Input: part model. Units: mm. Frame: model coordinates. Face numbers are marked on the shaded views. A direction names the side the tool comes from. Round coordinates to 2 decimals unless told otherwise and drop trailing zeros. Write each loop counter-clockwise with the first axis right and the second up, starting at its lowest first coordinate (ties: lowest second). Pieces come first, ordered by that corner, then holes. Notation, with made-up numbers: (38.5, -23) -> (44.5, -23) arc R26 ccw to (44.5, 7) -> close; hole circle Ø11 at (58.25, 12.25). An arc over 180 degrees is marked (long way). Write item = value, one per line.
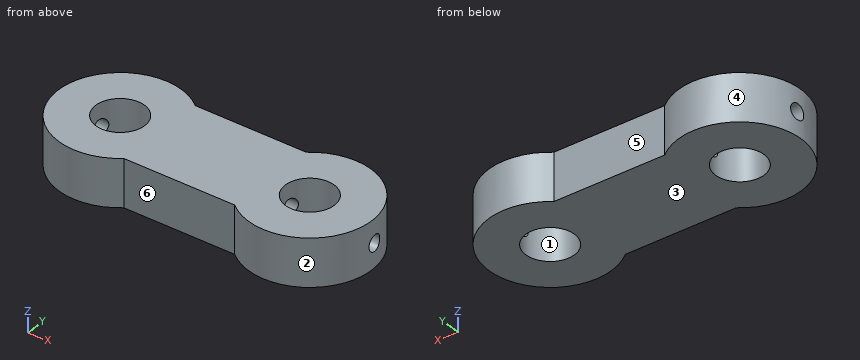
Autodesk Fusion 360 part; units mm, degrees
sketch "Eskiz1" plane through (0, 0, 0) normal (0, 0, 1) x (1, 0, 0)
  circle A0 centre (0, 0) radius 5.15
  circle A1 centre (40, 0) radius 5.15
  line L0 (8.3066, 10) -> (31.6934, 10)
  line L1 (20, -10) -> (8.3066, -10)
  line L2 (20, -10) -> (31.6934, -10)
  arc A2 (8.3066, 10) -> (8.3066, -10) centre (0, 0) ccw
  arc A3 (31.6934, -10) -> (31.6934, 10) centre (40, 0) ccw
  dimension "d1" = 26
  dimension "d2" = 40
  dimension "d3" = 26
  dimension "d4" = 10.3
  dimension "d5" = 10.3
extrude "Ekstrüde Et1" add sketch "Eskiz1" along normal blind 10 makes body 1
sketch "Eskiz2" plane through (0, 0, 0) normal (0, 0, 1) x (1, 0, 0)
  line L0 (-25, 0) -> (-24, 0)
  line L1 (-24, 0) -> (-24, 2)
  line L2 (-24, 2) -> (-25, 2)
  line L3 (-25, 2) -> (-25, 0)
extrude "Ekstrüde Et2" add sketch "Eskiz2" along normal blind 5 separate body makes body 2
sketch "Eskiz3" plane through (-25, 0, 0) normal (-1, 0, 0) x (0, -1, 0)
  line L0 (-2, 0) -> (0, 0)
  line L1 (0, 0) -> (0, 5)
  line L2 (0, 5) -> (-2, 5)
  line L3 (-2, 5) -> (-2, 0)
  line L4 (-1, 5) -> (-1, 4.2255)
hole "Delik1" at (-25, 1, 5) direction (1, 0, 0) diameter 3.332 depth 80 tip angle 118 bodies 1 2
delete_body "GövdeyiKaldır1" bodies 2
equation "d1 = 10 mm + 16 mm"
equation "d3 = 16 mm + 10 mm"
1) Cut plane B-B (z = 5). Return the cut outline in (x, y).
Solutions:
outline = (-12.98, -0.67) arc R13 ccw to (8.31, -10) -> (31.69, -10) arc R13 ccw to (52.98, -0.67) -> (45.11, -0.67) arc R5.15 cw to (34.89, -0.67) -> (5.11, -0.67) arc R5.15 cw to (-5.11, -0.67) -> close; (-12.72, 2.67) -> (-4.41, 2.67) arc R5.15 cw to (4.41, 2.67) -> (35.59, 2.67) arc R5.15 cw to (44.41, 2.67) -> (52.72, 2.67) arc R13 ccw to (31.69, 10) -> (8.31, 10) arc R13 ccw to start
2) Draft query along Y for the marked faces 1, 2 and 3. Return one class per face: +Y half, -Y half, draft (parallel to the pull), parting line (faces both ways), or undercut.
Solutions:
face_1 = undercut
face_2 = parting line
face_3 = draft
3) Cut plane D-D (y = 0). Return the cut outline in (x, z), and give its area (3 significant figures).
Solutions:
outline = (-13, 0) -> (-5.15, 0) -> (-5.15, 3.67) -> (-13, 3.67) -> close; (-13, 6.33) -> (-5.15, 6.33) -> (-5.15, 10) -> (-13, 10) -> close; (5.15, 0) -> (34.85, 0) -> (34.85, 3.67) -> (5.15, 3.67) -> close; (5.15, 6.33) -> (34.85, 6.33) -> (34.85, 10) -> (5.15, 10) -> close; (45.15, 0) -> (53, 0) -> (53, 3.67) -> (45.15, 3.67) -> close; (45.15, 6.33) -> (53, 6.33) -> (53, 10) -> (45.15, 10) -> close
area = 333 mm^2
4) Cut plane A-A (x = 40). Return the cut outline in (y, z).
Solutions:
outline = (-13, 0) -> (-5.15, 0) -> (-5.15, 10) -> (-13, 10) -> close; (5.15, 0) -> (13, 0) -> (13, 10) -> (5.15, 10) -> close
5) Access query for the marked faces 4, 5 and 6. Directions: +Z, -Z, +X, -X, +Y, -Y. A direction counts if a zero-diameter tool reaches every point of the face in a straight line with its end or side. Return the directions, or none.
Solutions:
face_4 = +Z, -Z
face_5 = +Z, -Z, +Y
face_6 = +Z, -Z, -Y
6) Cut plane C-C (x = 10). Return the cut outline in (y, z).
Solutions:
outline = (-10, 0) -> (10, 0) -> (10, 10) -> (-10, 10) -> close; hole circle Ø3.33 at (1, 5)
7) First-contact query: P1, Ø1.5, axis at y = -2, z = 4, coming from the -X side; P2, Ø3, axis at y = 9.5, z = 8.5, coming from the -X side; P3, Ø2, axis at y = 5.5, z = 3.5, coming from the -X side. Flat tips, straight axial feed; report the tip coordinate or a pass-through.
Solutions:
P1 = -12.94
P2 = -10.25
P3 = -12.2
8) Line query: L1, parallel to X at y = 0, z = 2.75; L2, parallel to Z at x = -9.5, y = 1; L3, parallel to Y at x = 0, z = 4.75. Output: solid intervals per line, ascending. Write a range as from..to.
Solutions:
L1 = -13..-5.15, 5.15..34.85, 45.15..53
L2 = 0..3.33, 6.67..10
L3 = -13..-5.15, 5.15..13
